from build123d import *

# Parameters (mm, degrees)
SKETCH_1_W          = 270
SKETCH_1_H          = 210
EXTRUDE_1_DEPTH     = 3
SKETCH_2_R          = 2.15
CUT_EXTRUDE_1_DEPTH = 3
CUT_EXTRUDE_2_DEPTH = 10
SKETCH_4_W          = 20
SKETCH_4_H          = 15
CUT_EXTRUDE_3_DEPTH = 10
SKETCH_5_R          = 1.3
SKETCH_5_R_2        = 1.6
SKETCH_5_W          = 30
SKETCH_5_H          = 10
CUT_EXTRUDE_4_DEPTH = 10
CUT_EXTRUDE_5_DEPTH = 10
SKETCH_7_W          = 50
SKETCH_7_H          = 40
CUT_EXTRUDE_6_DEPTH = 10
FILLET_1_R          = 2


with BuildPart() as part:
    # 草图1 → 凸台-拉伸1 (new body)
    with BuildSketch(Plane(origin=(0, 0, 0), x_dir=(1, 0, 0), z_dir=(0, 1, 0))):
        Rectangle(SKETCH_1_W, SKETCH_1_H)
    extrude(amount=EXTRUDE_1_DEPTH)

    # 草图2 → 切除-拉伸1 (cut)
    with BuildSketch(Plane(origin=(0, 3, 0), x_dir=(1, 0, 0), z_dir=(0, 1, 0))):
        with Locations(Location((-100, 75, 0), (0, 0, 270))):
            Circle(SKETCH_2_R)
        with Locations(Location((100, 75, 0), (0, 0, 270))):
            Circle(SKETCH_2_R)
        with Locations(Location((100, -75, 0), (0, 0, 270))):
            Circle(SKETCH_2_R)
        with Locations(Location((-100, -75, 0), (0, 0, 270))):
            Circle(SKETCH_2_R)
    extrude(amount=-CUT_EXTRUDE_1_DEPTH, mode=Mode.SUBTRACT)

    # 草图3 → 切除-拉伸2 (cut)
    with BuildSketch(Plane(origin=(0, 3, 0), x_dir=(1, 0, 0), z_dir=(0, 1, 0))):
        with BuildLine():
            Line((-77.5, -80.3), (-76.5, -80.3))
            ThreePointArc((-76.5, -80.3), (-74.3, -82.5), (-76.5, -84.7))
            Line((-76.5, -84.7), (-77.5, -84.7))
            ThreePointArc((-77.5, -84.7), (-79.7, -82.5), (-77.5, -80.3))
        make_face()
        with BuildLine():
            Line((-62.5, -80.3), (-63.5, -80.3))
            ThreePointArc((-63.5, -80.3), (-65.7, -82.5), (-63.5, -84.7))
            Line((-63.5, -84.7), (-62.5, -84.7))
            ThreePointArc((-62.5, -84.7), (-60.3, -82.5), (-62.5, -80.3))
        make_face()
        with BuildLine():
            Line((-77.5, -99.7), (-76.5, -99.7))
            ThreePointArc((-76.5, -99.7), (-74.3, -97.5), (-76.5, -95.3))
            Line((-76.5, -95.3), (-77.5, -95.3))
            ThreePointArc((-77.5, -95.3), (-79.7, -97.5), (-77.5, -99.7))
        make_face()
        with BuildLine():
            Line((-62.5, -99.7), (-63.5, -99.7))
            ThreePointArc((-63.5, -99.7), (-65.7, -97.5), (-63.5, -95.3))
            Line((-63.5, -95.3), (-62.5, -95.3))
            ThreePointArc((-62.5, -95.3), (-60.3, -97.5), (-62.5, -99.7))
        make_face()
        with BuildLine():
            Line((62.5, -99.7), (63.5, -99.7))
            ThreePointArc((63.5, -99.7), (65.7, -97.5), (63.5, -95.3))
            Line((63.5, -95.3), (62.5, -95.3))
            ThreePointArc((62.5, -95.3), (60.3, -97.5), (62.5, -99.7))
        make_face()
        with BuildLine():
            Line((77.5, -99.7), (76.5, -99.7))
            ThreePointArc((76.5, -99.7), (74.3, -97.5), (76.5, -95.3))
            Line((76.5, -95.3), (77.5, -95.3))
            ThreePointArc((77.5, -95.3), (79.7, -97.5), (77.5, -99.7))
        make_face()
        with BuildLine():
            Line((77.5, -80.3), (76.5, -80.3))
            ThreePointArc((76.5, -80.3), (74.3, -82.5), (76.5, -84.7))
            Line((76.5, -84.7), (77.5, -84.7))
            ThreePointArc((77.5, -84.7), (79.7, -82.5), (77.5, -80.3))
        make_face()
        with BuildLine():
            Line((62.5, -80.3), (63.5, -80.3))
            ThreePointArc((63.5, -80.3), (65.7, -82.5), (63.5, -84.7))
            Line((63.5, -84.7), (62.5, -84.7))
            ThreePointArc((62.5, -84.7), (60.3, -82.5), (62.5, -80.3))
        make_face()
        with BuildLine():
            Line((-77.5, 80.3), (-76.5, 80.3))
            ThreePointArc((-76.5, 80.3), (-74.3, 82.5), (-76.5, 84.7))
            Line((-76.5, 84.7), (-77.5, 84.7))
            ThreePointArc((-77.5, 84.7), (-79.7, 82.5), (-77.5, 80.3))
        make_face()
        with BuildLine():
            Line((-62.5, 80.3), (-63.5, 80.3))
            ThreePointArc((-63.5, 80.3), (-65.7, 82.5), (-63.5, 84.7))
            Line((-63.5, 84.7), (-62.5, 84.7))
            ThreePointArc((-62.5, 84.7), (-60.3, 82.5), (-62.5, 80.3))
        make_face()
        with BuildLine():
            Line((-77.5, 99.7), (-76.5, 99.7))
            ThreePointArc((-76.5, 99.7), (-74.3, 97.5), (-76.5, 95.3))
            Line((-76.5, 95.3), (-77.5, 95.3))
            ThreePointArc((-77.5, 95.3), (-79.7, 97.5), (-77.5, 99.7))
        make_face()
        with BuildLine():
            Line((-62.5, 99.7), (-63.5, 99.7))
            ThreePointArc((-63.5, 99.7), (-65.7, 97.5), (-63.5, 95.3))
            Line((-63.5, 95.3), (-62.5, 95.3))
            ThreePointArc((-62.5, 95.3), (-60.3, 97.5), (-62.5, 99.7))
        make_face()
        with BuildLine():
            Line((62.5, 99.7), (63.5, 99.7))
            ThreePointArc((63.5, 99.7), (65.7, 97.5), (63.5, 95.3))
            Line((63.5, 95.3), (62.5, 95.3))
            ThreePointArc((62.5, 95.3), (60.3, 97.5), (62.5, 99.7))
        make_face()
        with BuildLine():
            Line((77.5, 99.7), (76.5, 99.7))
            ThreePointArc((76.5, 99.7), (74.3, 97.5), (76.5, 95.3))
            Line((76.5, 95.3), (77.5, 95.3))
            ThreePointArc((77.5, 95.3), (79.7, 97.5), (77.5, 99.7))
        make_face()
        with BuildLine():
            Line((77.5, 80.3), (76.5, 80.3))
            ThreePointArc((76.5, 80.3), (74.3, 82.5), (76.5, 84.7))
            Line((76.5, 84.7), (77.5, 84.7))
            ThreePointArc((77.5, 84.7), (79.7, 82.5), (77.5, 80.3))
        make_face()
        with BuildLine():
            Line((62.5, 80.3), (63.5, 80.3))
            ThreePointArc((63.5, 80.3), (65.7, 82.5), (63.5, 84.7))
            Line((63.5, 84.7), (62.5, 84.7))
            ThreePointArc((62.5, 84.7), (60.3, 82.5), (62.5, 80.3))
        make_face()
    extrude(amount=-CUT_EXTRUDE_2_DEPTH, mode=Mode.SUBTRACT)

    # 草图4 → 切除-拉伸3 (cut)
    with BuildSketch(Plane(origin=(0, 3, 0), x_dir=(1, 0, 0), z_dir=(0, 1, 0))):
        with Locations((-69.133090168, -59.966909832)):
            Rectangle(SKETCH_4_W, SKETCH_4_H)
        with Locations((69.133090168, -59.966909832)):
            Rectangle(SKETCH_4_W, SKETCH_4_H)
        with Locations((69.133090168, 59.966909832)):
            Rectangle(SKETCH_4_W, SKETCH_4_H)
        with Locations((-69.133090168, 59.966909832)):
            Rectangle(SKETCH_4_W, SKETCH_4_H)
    extrude(amount=-CUT_EXTRUDE_3_DEPTH, mode=Mode.SUBTRACT)

    # 草图5 → 切除-拉伸4 (cut)
    with BuildSketch(Plane(origin=(0, 3, 0), x_dir=(1, 0, 0), z_dir=(0, 1, 0))):
        with Locations(Location((-64, 24.35, 0), (0, 0, 270))):
            Circle(SKETCH_5_R)
        with Locations(Location((-6, 24.35, 0), (0, 0, 270))):
            Circle(SKETCH_5_R)
        with Locations(Location((56, 24.5, 0), (0, 0, 270))):
            Circle(SKETCH_5_R)
        with Locations(Location((114, 24.5, 0), (0, 0, 270))):
            Circle(SKETCH_5_R)
        with Locations(Location((114, -24.5, 0), (0, 0, 270))):
            Circle(SKETCH_5_R)
        with Locations(Location((56, -24.5, 0), (0, 0, 270))):
            Circle(SKETCH_5_R)
        with Locations(Location((-6, -24.35, 0), (0, 0, 270))):
            Circle(SKETCH_5_R)
        with Locations(Location((-64, -24.35, 0), (0, 0, 270))):
            Circle(SKETCH_5_R)
        with Locations(Location((-28.75, 102, 0), (0, 0, 270))):
            Circle(SKETCH_5_R_2)
        with Locations(Location((28.75, 102, 0), (0, 0, 270))):
            Circle(SKETCH_5_R_2)
        with Locations(Location((28.75, 55, 0), (0, 0, 270))):
            Circle(SKETCH_5_R_2)
        with Locations(Location((-28.75, 55, 0), (0, 0, 270))):
            Circle(SKETCH_5_R_2)
        with Locations(Location((-128.258252147, 13.258252147, 0), (0, 0, 270))):
            Circle(SKETCH_5_R)
        with Locations(Location((-101.741747853, -13.258252147, 0), (0, 0, 270))):
            Circle(SKETCH_5_R)
        with Locations((0, 55)):
            Rectangle(SKETCH_5_W, SKETCH_5_H)
    extrude(amount=-CUT_EXTRUDE_4_DEPTH, mode=Mode.SUBTRACT)

    # 草图6 → 切除-拉伸5 (cut)
    with BuildSketch(Plane(origin=(0, 3, 0), x_dir=(1, 0, 0), z_dir=(0, 1, 0))):
        with BuildLine():
            Line((-65, 105), (-135, 105))
            Line((-135, 105), (-135, 35))
            ThreePointArc((-135, 35), (-114.497474683, 84.497474683), (-65, 105))
        make_face()
        with BuildLine():
            Line((-135, -105), (-135, -35))
            ThreePointArc((-135, -35), (-114.497474683, -84.497474683), (-65, -105))
            Line((-65, -105), (-135, -105))
        make_face()
        with BuildLine():
            Line((65, -105), (135, -105))
            Line((135, -105), (135, -35))
            ThreePointArc((135, -35), (114.497474683, -84.497474683), (65, -105))
        make_face()
        with BuildLine():
            Line((135, 105), (135, 35))
            ThreePointArc((135, 35), (114.497474683, 84.497474683), (65, 105))
            Line((65, 105), (135, 105))
        make_face()
    extrude(amount=-CUT_EXTRUDE_5_DEPTH, mode=Mode.SUBTRACT)

    # 草图7 → 切除-拉伸6 (cut)
    with BuildSketch(Plane(origin=(0, 3, 0), x_dir=(1, 0, 0), z_dir=(0, 1, 0))):
        with Locations((-35, 0)):
            Rectangle(SKETCH_7_W, SKETCH_7_H)
        with Locations((85, 0)):
            Rectangle(SKETCH_7_W, SKETCH_7_H)
    extrude(amount=-CUT_EXTRUDE_6_DEPTH, mode=Mode.SUBTRACT)

    # 圆角1
    fillet_1_edges = [part.edges().sort_by_distance(p)[0] for p in [
        (-59.133090168, 1.5, -52.466909832),
        (-79.133090168, 1.5, -52.466909832),
        (-79.133090168, 1.5, -67.466909832),
        (-59.133090168, 1.5, -67.466909832),
        (79.133090168, 1.5, -67.466909832),
        (79.133090168, 1.5, -52.466909832),
        (59.133090168, 1.5, -52.466909832),
        (59.133090168, 1.5, -67.466909832),
        (59.133090168, 1.5, 52.466909832),
        (79.133090168, 1.5, 52.466909832),
        (79.133090168, 1.5, 67.466909832),
        (59.133090168, 1.5, 67.466909832),
        (-79.133090168, 1.5, 67.466909832),
        (-79.133090168, 1.5, 52.466909832),
        (-59.133090168, 1.5, 52.466909832),
        (-59.133090168, 1.5, 67.466909832),
        (15, 1.5, -60),
        (15, 1.5, -50),
        (-15, 1.5, -50),
        (-15, 1.5, -60),
        (-60, 1.5, 20),
        (-60, 1.5, -20),
        (-10, 1.5, -20),
        (-10, 1.5, 20),
        (110, 1.5, -20),
        (110, 1.5, 20),
        (60, 1.5, 20),
        (60, 1.5, -20),
    ]]
    fillet(fillet_1_edges, radius=FILLET_1_R)


solid = part.part
Build history of the part. All positions in model axes, mm. Round coordinates to 2 decimals unless told otherwise and drop trailing zeros. Loops run counter-clockwise (first coordinate to the right, second up) from the corner with the lowest first, then second, coordinate; pieces in that order, holes last. Notation, with made-up numbers: (68, 46) -> (92, 46) arc R21 ccw to (92, 76) -> close; hole circle Ø7 at (68, 8). An arc over 180 degrees is marked (long way). Answer in a Markdown table with one row per item.
Item 1: Saw through at B-B (y = 2.35). State how many separate pieces and enclosed holes the cut face has, and give its area (3 significant figures).
Answers below:
| item | result |
|---|---|
| separate pieces | 1 |
| enclosed holes | 41 |
| area | 46,600 mm² |
Item 2: Pin check, flat tips, straight feed: pin 1 (2 mm diameter, centred on x = 56, z = -24.5, fed in from -Y); pin 2 (1 mm diameter, centred on y = 2, z = -50, fed in from +X); pin 3 (1.1 mm diameter, centred on x = -77, y = 1.5, fed in from -Z); pin 4 (1.1 mm diameter, centred on x = 77, y = 2, fed in from +Z). Stop position of each tip, or through.
Answers below:
| item | result |
|---|---|
| pin 1 | passes through |
| pin 2 | stops at x = 133.48 |
| pin 3 | stops at z = -104.06 |
| pin 4 | stops at z = 104.06 |
Item 3: Drill centre lines: L1, parallel to X at y = 2.05, z = 24.35; L2, parallel to Z at x = 114, y = 1.45; L3, parallel to X at y = 1.3, z = -2. Where is each one in solid material? Low to high. Write a range as [from, to].
Answers below:
| item | result |
|---|---|
| L1 | x = [-135, -65.3], [-62.7, -7.3], [-4.7, 54.71], [57.29, 112.71], [115.29, 135] |
| L2 | z = [-84.99, -25.8], [-23.2, 23.2], [25.8, 84.99] |
| L3 | x = [-135, -60], [-10, 60], [110, 135] |
Item 4: Saw through at A-A (z = -1). Write the cut outline in (x, y).
Answers below:
| item | result |
|---|---|
| outline | (-135, 0) -> (-60, 0) -> (-60, 3) -> (-135, 3) -> close; (-10, 0) -> (60, 0) -> (60, 3) -> (-10, 3) -> close; (110, 0) -> (135, 0) -> (135, 3) -> (110, 3) -> close |
